from build123d import *

# Parameters (mm, degrees)
F0_W     = 44.5
F0_H     = 29
F1_DEPTH = 25.4
F2_R     = 10
F3_SIZE  = 1


with BuildPart() as f1:
    # F0 (on Right) → F1 (new body)
    with BuildSketch(Plane.YZ):
        with BuildLine():
            ThreePointArc((-27.7348309755, -3.6565796257), (-28.7256107674, 1.6113392583), (-27.7348309755, 6.8792581423))
            Line((-27.7348309755, 6.8792581423), (-27.7348309755, 16.1113392583))
            Line((-27.7348309755, 16.1113392583), (-28.8986135274, 16.1113392583))
            Line((-28.8986135274, 16.1113392583), (-28.8986135274, -12.8886607417))
            Line((-28.8986135274, -12.8886607417), (-27.7348309755, -12.8886607417))
            Line((-27.7348309755, -12.8886607417), (-27.7348309755, -3.6565796257))
        make_face()
        with BuildLine():
            ThreePointArc((-27.7348309755, 6.8792581423), (-22.4068446652, 13.5828643035), (-14.2256107674, 16.1113392583))
            Line((-14.2256107674, 16.1113392583), (-27.7348309755, 16.1113392583))
            Line((-27.7348309755, 16.1113392583), (-27.7348309755, 6.8792581423))
        make_face()
        with BuildLine():
            Line((-27.7348309755, -12.8886607417), (-14.2256107674, -12.8886607417))
            ThreePointArc((-14.2256107674, -12.8886607417), (-22.4068446652, -10.360185787), (-27.7348309755, -3.6565796257))
            Line((-27.7348309755, -3.6565796257), (-27.7348309755, -12.8886607417))
        make_face()
        with BuildLine():
            Line((-14.2256107674, -12.8886607417), (-14.2256107674, 16.1113392583))
            ThreePointArc((-14.2256107674, 16.1113392583), (-22.4068446652, 13.5828643035), (-27.7348309755, 6.8792581423))
            Line((-27.7348309755, 6.8792581423), (-27.7348309755, -3.6565796257))
            ThreePointArc((-27.7348309755, -3.6565796257), (-22.4068446652, -10.360185787), (-14.2256107674, -12.8886607417))
        make_face()
        with BuildLine():
            Line((-27.7348309755, -3.6565796257), (-27.7348309755, 6.8792581423))
            ThreePointArc((-27.7348309755, 6.8792581423), (-28.7256107674, 1.6113392583), (-27.7348309755, -3.6565796257))
        make_face()
        with Locations((8.0243892326, 1.6113392583)):
            Rectangle(F0_W, F0_H)
    extrude(amount=F1_DEPTH)

    # F2
    f2_edges = [f1.edges().sort_by_distance(p)[0] for p in [
        (25.4, -28.898614, 1.611339),
        (0, -28.898614, 1.611339),
    ]]
    fillet(f2_edges, radius=F2_R)

    # F3
    f3_edges = [f1.edges().sort_by_distance(p)[0] for p in [
        (25.4, 5.687888, 16.111339),
        (25.4, 5.687888, -12.888661),
        (12.7, 30.274389, 16.111339),
        (12.7, 30.274389, -12.888661),
        (25.4, 30.274389, 1.611339),
        (0, 30.274389, 1.611339),
    ]]
    chamfer(f3_edges, length=F3_SIZE)


solid = f1.part
Work out the finished part from the listing and answer in its coordinate system (mm). Round coordinates to 2 decimals unless told otherwise and drop trailing zeros. Write each loop counter-clockwise with the first axis right and the second up, starting at its lowest first coordinate (ties: lowest second). Pieces come first, ordered by that corner, then holes. Notation, with made-up numbers: (5.5, 6) -> (28.5, 6) arc R26 cw to (28.5, 28) -> close; hole circle Ø6 at (21.25, 58.5). An arc over 180 degrees is marked (long way). Write each question's results on one line, items separated by ' | '.
Item 1: Flat-ended cylindrical pins translate along their axes: P1, Ø5, axis at x = 19, z = 9.5, coming from the -Y side; P2, Ø12, axis at y = -20.5, z = 9.5, coming from the +X side; P3, Ø1.5, axis at x = 19, z = 10.5, coming from the -Y side. Find the tip coordinate at first contact, or state that the pin passes through.
Result set:
P1: y = -28.84 | P2: x = 25.4 | P3: y = -28.48
Item 2: A cutting plane is placed at A-A, the plane z = 7.5. Determine the outline of the cut face in (x, y), plus the area to 3 significant figures.
Result set:
outline: (0, -18.9) arc R10 ccw to (10, -28.9) -> (15.4, -28.9) arc R10 ccw to (25.4, -18.9) -> (25.4, 29.27) -> (24.4, 30.27) -> (1, 30.27) -> (0, 29.27) -> close | area: 1,460 mm^2
Item 3: Find the intervals of material crossed by line 1 along Y through (x, z) = (15.75, 2); line 2 along Y through (x, z) = (8, -2.5); line 3 along X through (y, z) = (-24.5, 2.5), in increasing order. Write a range as [from, to].
Result set:
line 1: [-28.89, 30.27] | line 2: [-28.7, 30.27] | line 3: [1.72, 23.68]
